Autodesk Inventor part; units mm, degrees
ref_plane "YZ Plane" through (0, 0, 0) normal (1, 0, 0) x (0, 1, 0)
ref_plane "XZ Plane" through (0, 0, 0) normal (0, 1, 0) x (-1, 0, 0)
ref_plane "XY Plane" through (0, 0, 0) normal (0, 0, 1) x (1, 0, 0)
sketch "Szkic2" plane through (0, 0, 0) normal (1, 0, 0) x (0, 1, 0)
  line L0 (-10.1243, 0) -> (60.0207, 0)
  line L1 (0, -10.1243) -> (0, 60.0207)
  line L2 (0, 20) -> (0, 0.5)
  line L3 (0.5, 0) -> (40, 0)
  line L4 (40, 2) -> (2.5, 2)
  line L5 (2, 2.5) -> (2, 20)
  line L6 (2, 20) -> (0, 20)
  line L7 (40, 0) -> (40, 2)
  arc A0 (2, 2.5) -> (2.5, 2) centre (2.5, 2.5) ccw
  arc A1 (0, 0.5) -> (0.5, 0) centre (0.5, 0.5) ccw
  point P0 (0, 0)
  point P1 (0, 0)
  dimension "d4" = 2
  dimension "d5" = 2
  dimension "d6" = 40
  dimension "d7" = 20
  dimension "d8" = 0.5
extrude "Wyciągnięcie proste1" add sketch "Szkic2" along normal blind 15 contours A1 L1 L6 L5 A0 L4 L7 L0
sketch "Szkic3" plane through (0, 0, 0.5) normal (0, -1, 0) x (1, 0, 0)
  circle A0 centre (7.5, 15) radius 1
  point P0 (0, -0.5)
  dimension "d11" = 2
hole "Otwór1" at (7.5, 0, 15.5) direction (0, 1, 0) diameter 2 end through all
properties part number "kątownik_bloczek"
Can you work these out from the model? Positions are in its coordinate system, mm. A direction names the side the tool comes from. Round coordinates to 2 decimals unless told otherwise and drop trailing zeros. Write each loop counter-clockwise with the first axis right and the second up, starting at its lowest first coordinate (ties: lowest second). Pieces come first, ordered by that corner, then holes. Notation, with made-up numbers: (77, 30) - (87, 30) arc R21 cw to (87, 56) - close; hole circle Ø8 at (-39, 73.25). An arc over 180 degrees is marked (long way). Write each question's results on one line, items separated by ' | '. Start each with the question number.
1) We'd pull the mould along X, two halves only. Please class faces 1 (the flat face through (7, 2, 11)), 2 (the flat face through (0, 14, 1)), 3 (the cylindrical face through (7.2, 1.014, 14.546)): released by +X, released by -X, zero draft, split by the parting line, or undercut.
2) Suppose I cut it at B-B (x = 10). List the corners of the cut face in (y, z) for me.
3) Which directions (+Z, -Z, +X, -X, +Y, -Y) give clear straight access to the entire face, cutting with the end or side of a thin tool? Please do faces 4 (the flat face through (7, 40, 1)), 5 (the flat face through (7, 22, 2)).
4) Suppose I cut it at A-A (z = 15.5). List the corners of the cut face in (x, y) for me.
5) Suppose I cut it at C-C (y = 16). List the corners of the cut face in (x, z) for me, and give its area (3 significant figures).
6) Please list where these lines run through material, in increasing order: line 1 (Z direction, x = 7.5, y = 1.2); line 2 (X direction, y = 0.4, z = 15.5); line 3 (Z direction, x = 10, y = 7).
7) For pin 1 Ø1.5 at (x, z) = (3, 11) entering from +Y, with a flat end and sliding along its axis, tell me the tip position at first contact or that it passes through.
Here are the results:
1) face 1: zero draft | face 2: released by -X | face 3: undercut
2) outline: (0, 0.5) arc R0.5 ccw to (0.5, 0) - (40, 0) - (40, 2) - (2.5, 2) arc R0.5 cw to (2, 2.5) - (2, 20) - (0, 20) - close
3) face 4: +Z, -Z, +X, -X, +Y | face 5: +Z, +X, -X, +Y
4) outline: (0, 0) - (6.5, 0) - (6.5, 2) - (0, 2) - close; (8.5, 0) - (15, 0) - (15, 2) - (8.5, 2) - close
5) outline: (0, 0) - (15, 0) - (15, 2) - (0, 2) - close | area: 30.0 mm2
6) line 1: z = 0 to 14.5, 16.5 to 20 | line 2: x = 0 to 6.5, 8.5 to 15 | line 3: z = 0 to 2
7) pin 1: stops at y = 2
